Autodesk Inventor part; units mm, degrees
ref_plane "YZ Plane" through (0, 0, 0) normal (1, 0, 0) x (0, 1, 0)
ref_plane "XZ Plane" through (0, 0, 0) normal (0, 1, 0) x (-1, 0, 0)
ref_plane "XY Plane" through (0, 0, 0) normal (0, 0, 1) x (1, 0, 0)
sketch "Sketch1" plane through (0, 0, 0) normal (0, 0, 1) x (1, 0, 0)
  circle A0 centre (0, 0) radius 1.55
  line L0 (0, 0) -> (30.548, 0)
  circle A1 centre (30.548, 0) radius 1.55
  line L1 (30.548, 0) -> (51.3166, -5.9278)
  circle A2 centre (51.3166, -5.9278) radius 1.55
  line L2 (0, 0) -> (-5, 0)
  line L3 (-5, 0) -> (-5, 6)
  line L4 (-5, 6) -> (1.9282, 10)
  line L5 (-5, 0) -> (-5, -6)
  line L6 (1.9282, 10) -> (30.548, 10)
  line L7 (-5, -6) -> (1.9282, -10)
  line L8 (1.9282, -10) -> (30.548, -10)
  line L9 (30.548, -10) -> (49.4624, -15.3986)
  line L10 (30.548, 10) -> (53.1707, 3.5429)
  line L11 (0, 0) -> (1.9282, 0)
  line L12 (51.3166, -5.9278) -> (75.3565, -12.7894)
  line L13 (75.3565, -12.7894) -> (76.4544, -8.943)
  line L14 (76.4544, -8.943) -> (53.1707, 3.5429)
  line L15 (75.3565, -12.7894) -> (74.2587, -16.6358)
  line L16 (49.4624, -15.3986) -> (74.2587, -16.6358)
  line L17 (51.3166, -5.9278) -> (75.3565, -12.7894)
  circle A3 centre (63.3366, -9.3586) radius 1.5
  line L18 (63.3366, -9.3586) -> (71.0293, -11.5543)
  circle A4 centre (71.0293, -11.5543) radius 1.5
  dimension "d0" = 3.1
  dimension "d1" = 30.548
  dimension "d2" = 3.1
  dimension "d3" = 164.07
  dimension "d4" = 3.1
  dimension "d5" = 21.598
  dimension "d6" = 5
  dimension "d7" = 6
  dimension "d8" = 6
  dimension "d9" = 120
  dimension "d10" = 8
  dimension "d11" = 120
  dimension "d12" = 8
  dimension "d13" = 28.6198
  dimension "d14" = 28.6198
  dimension "d15" = 19.6698
  dimension "d16" = 23.5262
  dimension "d23" = 1.9282
  dimension "d54" = 25
  dimension "d55" = 180
  dimension "d56" = 4
  dimension "d57" = 4
  dimension "d58" = 90
  dimension "d59" = 90
  dimension "d60" = 3
  dimension "d61" = 8
  dimension "d62" = 3
extrude "Extrusion1" add sketch "Sketch1" along normal blind 4 contours L0 A1 L1 A2 L12 A3 A4 L15 L16 L9 L8 L7 L5 L2 A0 | A0 L2 L3 L4 L6 L10 L14 L13 L12 A4 A3 A2 L1 A1 L0
sketch "Sketch3" plane through (0, 0, 4) normal (0, 0, 1) x (1, 0, 0)
  line L0 (1.9282, -10) -> (30.548, -10)
  line L1 (30.548, -10) -> (49.4624, -15.3986)
  line L2 (49.4624, -15.3986) -> (74.2587, -16.6358)
  line L3 (74.2587, -16.6358) -> (76.4544, -8.943)
  line L4 (76.4544, -8.943) -> (53.1707, 3.5429)
  line L5 (53.1707, 3.5429) -> (30.548, 10)
  line L6 (30.548, 10) -> (1.9282, 10)
  line L7 (1.9282, 10) -> (-5, 6)
  line L8 (-5, 6) -> (-5, -6)
  line L9 (-5, -6) -> (1.9282, -10)
  circle A0 centre (71.0293, -11.5543) radius 1.5
  circle A1 centre (63.3366, -9.3586) radius 1.5
  circle A2 centre (51.3166, -5.9278) radius 1.55
  circle A3 centre (30.548, 0) radius 1.55
  circle A4 centre (0, 0) radius 1.55
  line L10 (49.4624, -15.3986) -> (42.7525, -7.984)
  line L11 (42.7525, -7.984) -> (43.8857, -0.1703)
  line L12 (43.8857, -0.1703) -> (53.1707, 3.5429)
  dimension "d63" = 10
  dimension "d64" = 10
  dimension "d65" = 130
  dimension "d66" = 135
extrude "Extrusion2" add sketch "Sketch3" against normal blind 7 contours L10 L11 L12 L4 L3 L2
sketch "Sketch4" plane through (0, 0, -3) normal (0, 0, -1) x (-1, 0, 0)
  line L0 (-53.1707, 3.5429) -> (-76.4544, -8.943)
  line L1 (-76.4544, -8.943) -> (-74.2587, -16.6358)
  line L2 (-74.2587, -16.6358) -> (-49.4624, -15.3986)
  line L3 (-49.4624, -15.3986) -> (-42.7525, -7.984)
  line L4 (-42.7525, -7.984) -> (-43.8857, -0.1703)
  line L5 (-43.8857, -0.1703) -> (-53.1707, 3.5429)
  circle A0 centre (-71.0293, -11.5543) radius 1.5
  circle A1 centre (-51.3166, -5.9278) radius 1.55
  circle A2 centre (-63.3366, -9.3586) radius 1.5
  circle A3 centre (-71.0293, -11.5543) radius 2.8
  circle A4 centre (-63.3366, -9.3586) radius 2.8
  circle A5 centre (-51.3166, -5.9278) radius 2.8
  point P0 (0, 0)
  dimension "d69" = 5.6
  dimension "d70" = 5.6
  dimension "d71" = 5.6
extrude "Extrusion3" cut sketch "Sketch4" against normal blind 2 contours A3 | A4 | A5
chamfer "Chamfer1" distance 2 angle 45 10 edges at (41.8594, 6.7715, 0) (16.2381, -10, 0) (40.0052, -12.6993, 0) (-1.5359, -8, 0) (-5, 0, 0) (-1.5359, 8, 0) (16.2381, 10, 0) (48.5282, 1.6863, -3) (43.3191, -4.0771, -3) (46.1075, -11.6913, -3)
equation "\"d8\" = d7"
equation "\"d11\" = d9"
equation "\"d12\" = d10"
equation "\"d13\" = d1 - d23"
equation "\"d14\" = d1 - d23"
equation "\"d15\" = d5 - d23"
equation "\"d16\" = d5 + d23"
equation "\"d57\" = d56"
equation "\"d58\" = d59"
equation "\"d70\" = d69"
equation "\"d71\" = d69"
properties part number "Fibula"
Design review of the part built by this model. Coordinates are the model's own, in mm. A direction names the side the tool comes from. Coordinates: 2 decimals unless noted, no trailing zeros. Order: outer loops, then holes, each group sorted by start corner. A loop starts at its lowest first (then second) coordinate and runs counter-clockwise, first axis right, second up. Notation, with made-up numbers: (22.5, -13) - (81.5, -13) arc R28 cw to (81.5, 21) - close; hole circle Ø5 at (36, 86.5). An arc over 180 degrees is marked (long way). Answer in a Markdown table with one row per item.
(1) Consider section D-D on x = 57. State the section outline as (y, z) points.
Checked values:
| item | result |
|---|---|
| outline | (-15.77, -3) - (1.49, -3) - (1.49, 4) - (-15.77, 4) - close |
(2) Wall thickness on line 1 along X through (y, z) = (0, 1.15); line 2 along X through (y, z) = (0, 3.05); line 3 along Z through (x, y) = (4, 6.5): over which ranges is each line inside the solid? List them lowest first. Write a range as from..to.
Checked values:
| item | result |
|---|---|
| line 1 | -4.15..-1.55, 1.55..29, 32.1..59.78 |
| line 2 | -5..-1.55, 1.55..29, 32.1..59.78 |
| line 3 | 0..4 |
(3) For faces 1 (the flat face through (-5, 0, 3)), 2 (the flat face through (70, -13, -1)), 3 (the flat face through (46.9, -12.57, -0.48)), list the 3-axis set-ups (+Z, -Z, +X, -X, +Y, -Y) from which the entire face can be reached by the end or side of a thin tool; tool diameter is ignored.
Checked values:
| item | result |
|---|---|
| face 1 | +Z, -Z, -X, +Y, -Y |
| face 2 | -Z |
| face 3 | -Z, -X, -Y |
(4) Clearance check with flat-ended pins moving along their axes: pin 1 (1 mm diameter, centred on x = 18, z = 3, fed in from -Y); pin 2 (1.5 mm diameter, centred on x = 62, z = -0.5, fed in from -Y); pin 3 (4.5 mm diameter, centred on x = 71.03, y = -11.55, fed in from -Z). State where each tip first meets the part, or that it passes through.
Checked values:
| item | result |
|---|---|
| pin 1 | y = -10 |
| pin 2 | y = -16.06 |
| pin 3 | z = -1 |
(5) Consider section A-A on x = 0. State the section outline as (y, z) points, plus the area to 3 significant figures.
Checked values:
| item | result |
|---|---|
| outline | (-8.89, 2) - (-6.58, 0) - (-1.55, 0) - (-1.55, 4) - (-8.89, 4) - close; (1.55, 0) - (6.58, 0) - (8.89, 2) - (8.89, 4) - (1.55, 4) - close |
| area | 54.1 mm^2 |
(6) The part is to be moulded in two halves that separate along Y. For faces 4 (the flat face through (62, -11, -1)), 5 (the flat face through (16, -10, 3)), 6 (the flat face through (-4, 0, 1)), say which applies: released by +Y, released by -Y, zero draft, split by the parting line, or undercut.
Checked values:
| item | result |
|---|---|
| face 4 | undercut |
| face 5 | released by -Y |
| face 6 | zero draft |
(7) Consider section C-C on x = 24. State the section outline as (y, z) points, plus the area to 3 significant figures.
Checked values:
| item | result |
|---|---|
| outline | (-10, 2) - (-8, 0) - (8, 0) - (10, 2) - (10, 4) - (-10, 4) - close |
| area | 76.0 mm^2 |
(8) Consider section B-B on z = 1. State the section outline as (x, y) points.
Checked values:
| item | result |
|---|---|
| outline | (-4, -5.42) - (2.2, -9) - (30.69, -9) - (48.19, -14) - (49.46, -15.4) - (74.26, -16.64) - (76.45, -8.94) - (53.17, 3.54) - (51.65, 2.94) - (30.41, 9) - (2.2, 9) - (-4, 5.42) - close; hole circle Ø3.1 at (0, 0); hole circle Ø3.1 at (30.55, 0); hole circle Ø3.1 at (51.32, -5.93); hole circle Ø3 at (63.34, -9.36); hole circle Ø3 at (71.03, -11.55) |
